Geometry check sheet. Reference: drawing and pictorial views, mm from the part's lowest x, y, z. Coordinates: 2 decimals unless noted, no trailing zeros. Loops run counter-clockwise (first coordinate to the right, second up) from the corner with the lowest first, then second, coordinate; pieces in that order, holes last. Notation, with made-up numbers: (73, 1) - (128, 1) arc R23 ccw to (128, 14) - close; hole circle Ø8 at (56, 83). An arc over 180 degrees is marked (long way). One line per item, written item: value.
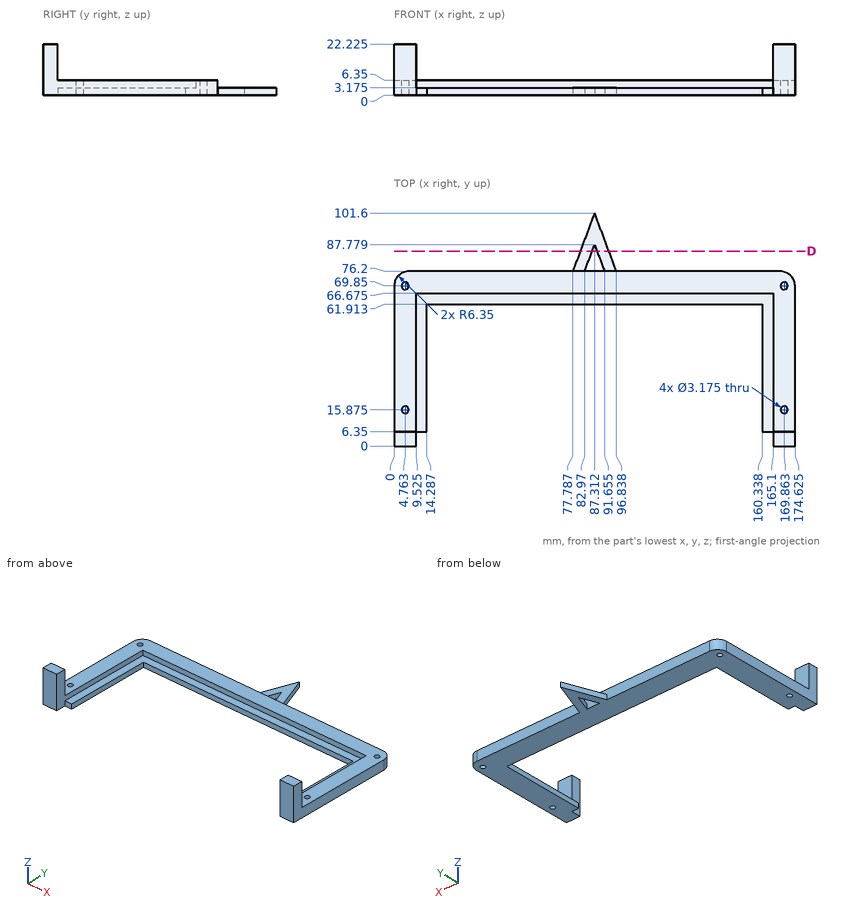
(1) Go/stop test with flat-tipped pins: pin 1 Ø2.5 at (x, y) = (4.76, 15.88) entering from -Z; pin 2 Ø3.5 at (x, z) = (78.5, 2.5) entering from -Y; pin 3 Ø9.5 at (x, y) = (83.5, 93) entering from +Z (1 decimal); pin 4 Ø1.6 at (x, z) = (162, 2) entering from -Y. Record where each tip stops, or that it passes through.
Reply:
pin 1: through
pin 2: y = 61.91
pin 3: z = 3.2
pin 4: y = 6.35
(2) Cross-section at D-D on y = 85. Record the cut outline in (x, z) (1 decimal), and give its area (3 significant figures).
Reply:
outline: (81.1, 0) - (86.3, 0) - (86.3, 3.2) - (81.1, 3.2) - close; (88.4, 0) - (93.5, 0) - (93.5, 3.2) - (88.4, 3.2) - close
area: 32.9 mm2
(3) Material ranges on probe 1 along X at (y, z) = (10.5, 1.25) (1 decimal); probe 2 along X at (y, z) = (24, 6) (1 decimal); probe 3 along Y at (x, z) = (118.5, 6.25) (1 decimal), recorded low to high. Write a range as from..to.
Reply:
probe 1: 0..14.3, 160.3..174.6
probe 2: 0..9.5, 165.1..174.6
probe 3: 66.7..76.2
